Autodesk Inventor part; units mm, degrees
ref_plane "YZ Plane" through (0, 0, 0) normal (1, 0, 0) x (0, 1, 0)
ref_plane "XZ Plane" through (0, 0, 0) normal (0, 1, 0) x (-1, 0, 0)
ref_plane "XY Plane" through (0, 0, 0) normal (0, 0, 1) x (1, 0, 0)
sketch "Skizze1" plane through (0, 0, 0) normal (0, 0, 1) x (1, 0, 0)
  arc A0 (-10.0563, 3.3011) -> (-12.2178, -3.2473) centre (-1.2178, -3.2473) ccw
  line L0 (-12.2178, -3.2473) -> (9.7822, -3.2473)
  arc A1 (9.7822, -3.2473) -> (7.6207, 3.3011) centre (-1.2178, -3.2473) ccw
  arc A2 (-3.7041, 1.8719) -> (7.6207, 3.3011) centre (-1.2178, 27.7527) ccw
  line L1 (-3.7041, 1.8719) -> (-4.2446, 1.7527)
  line L2 (-4.2446, 1.7527) -> (-4.7816, 1.7527)
  line L3 (-4.7816, 1.7527) -> (-6.4898, 2.2928)
  arc A3 (-10.0563, 3.3011) -> (-6.4898, 2.2928) centre (-1.2178, 27.7527) ccw
  arc A4 (-12.2178, 58.7527) -> (-10.0563, 52.2043) centre (-1.2178, 58.7527) ccw
  arc A5 (7.6207, 52.2043) -> (-10.0563, 52.2043) centre (-1.2178, 27.7527) ccw
  arc A6 (7.6207, 52.2043) -> (9.7822, 58.7527) centre (-1.2178, 58.7527) ccw
  line L4 (9.7822, 58.7527) -> (-12.2178, 58.7527)
  line L5 (85.2075, 58.7527) -> (80.2075, 58.7527)
  line L6 (80.2075, 58.7527) -> (80.2075, 53.7527)
  line L7 (80.2075, 53.7527) -> (85.2075, 53.7527)
  line L8 (85.2075, 53.7527) -> (85.2075, 58.7527)
  line L9 (85.2075, -3.2473) -> (85.2075, 1.7527)
  line L10 (85.2075, 1.7527) -> (80.2075, 1.7527)
  line L11 (80.2075, 1.7527) -> (80.2075, -3.2473)
  line L12 (80.2075, -3.2473) -> (85.2075, -3.2473)
  circle A7 centre (19.8794, 52.7527) radius 3
  circle A8 centre (19.8794, 2.7527) radius 3
  circle A9 centre (-22.1206, 2.7527) radius 3
  circle A10 centre (-22.1206, 52.7527) radius 3
  line L13 (85.2075, 58.7527) -> (-62.1847, 58.7527)
  line L14 (-62.1847, 58.7527) -> (-62.1847, -3.2473)
  line L15 (-62.1847, -3.2473) -> (85.2075, -3.2473)
  line L16 (85.2075, -3.2473) -> (85.2075, 58.7527)
  point P0 (0, 0)
extrude "Extrusion1" add sketch "Skizze1" along normal blind 3
sketch "Skizze2" plane through (0, 0, 3) normal (0, 0, 1) x (1, 0, 0)
  circle A0 centre (-3.1206, 27.7527) radius 15
  line L0 (85.2075, 58.7527) -> (-62.1847, 58.7527)
  line L1 (-62.1847, -3.2473) -> (85.2075, -3.2473)
  line L2 (27.3951, 58.7527) -> (31.3951, 58.7527)
  line L3 (31.3951, 58.7527) -> (31.3951, -3.2473)
  line L4 (31.3951, -3.2473) -> (27.3951, -3.2473)
  line L5 (27.3951, -3.2473) -> (27.3951, 58.7527)
  line L6 (35.5129, 58.7527) -> (39.5129, 58.7527)
  line L7 (39.5129, 58.7527) -> (39.5129, 3.8427)
  line L8 (39.5129, 3.8427) -> (35.5129, 3.8427)
  line L9 (35.5129, 3.8427) -> (35.5129, 58.7527)
  line L10 (85.2075, -3.2473) -> (85.2075, 58.7527)
  line L11 (39.5129, 3.8427) -> (85.2075, 3.8427)
  line L12 (85.2075, 3.8427) -> (85.2075, 7.8427)
  line L13 (85.2075, 7.8427) -> (39.5129, 7.8427)
  line L14 (39.5129, 7.8427) -> (39.5129, 3.8427)
  line L15 (39.5129, 58.7527) -> (85.2075, 58.7527)
  line L16 (85.2075, 58.7527) -> (85.2075, 54.7527)
  line L17 (85.2075, 54.7527) -> (39.5129, 54.7527)
  line L18 (39.5129, 54.7527) -> (39.5129, 58.7527)
  point P0 (0, 0)
  dimension "d2" = 4
  dimension "d3" = 4
  dimension "d4" = 45.6946
  dimension "d5" = 4
  dimension "d12" = 45.6946
  dimension "d13" = 4
extrude "Extrusion2" add sketch "Skizze2" along normal blind 35 contours L10 L17 L7 L0 | L7 L8 L9 L0 | L10 L11 L7 L13 | L3 L1 L5 L0
sketch "Skizze3" plane through (0, 0, 3) normal (0, 0, 1) x (1, 0, 0)
  line L0 (39.5129, 54.7527) -> (39.5129, 7.8427)
  line L1 (39.5129, 7.8427) -> (85.2075, 7.8427)
  line L2 (85.2075, 7.8427) -> (85.2075, 54.7527)
  line L3 (35.5129, 58.7527) -> (31.3951, 58.7527)
  line L4 (27.7822, 53.7527) -> (85.2075, 53.7527)
  line L5 (39.5129, 7.8427) -> (85.2075, 7.8427)
  line L6 (85.2075, 7.8427) -> (85.2075, 53.7527)
  line L7 (85.2075, 53.7527) -> (39.5129, 53.7527)
  line L8 (39.5129, 53.7527) -> (39.5129, 7.8427)
  line L9 (35.5129, 3.8427) -> (35.5129, 58.7527)
  line L10 (31.3951, 58.7527) -> (31.3951, -3.2473)
  line L11 (31.3951, -3.2473) -> (85.2075, -3.2473)
  line L12 (85.2075, -3.2473) -> (85.2075, 3.8427)
  line L13 (85.2075, 3.8427) -> (35.5129, 3.8427)
  line L14 (85.2075, 54.7527) -> (39.5129, 54.7527)
  line L15 (27.3951, -3.2473) -> (27.3951, 58.7527)
  line L16 (27.3951, 58.7527) -> (-62.1847, 58.7527)
  line L17 (-62.1847, 58.7527) -> (-62.1847, -3.2473)
  line L18 (-62.1847, -3.2473) -> (27.3951, -3.2473)
  point P0 (0, 0)
extrude "Extrusion3" cut sketch "Skizze3" against normal blind 35 contours L4 L2 L1 L0
sketch "Skizze4" plane through (39.5129, 7.8427, 38) normal (1, 0, 0) x (0, 0, -1)
  line L0 (0, 0) -> (38, 0)
  line L1 (38, 45.91) -> (38, 0)
  line L2 (35, 45.91) -> (38, 45.91)
  line L3 (35, 46.91) -> (35, 45.91)
  line L4 (0, 0) -> (0, 46.91)
  line L5 (0, 0) -> (38, 0)
  line L6 (33.1404, 0) -> (3.7306, 0)
  line L7 (3.7306, 0) -> (3.7306, 42.1415)
  line L8 (3.7306, 42.1415) -> (33.1404, 42.1415)
  line L9 (33.1404, 42.1415) -> (33.1404, 0)
  line L10 (35, 46.91) -> (0, 46.91)
  point P0 (38, -7.8427)
extrude "Extrusion4" cut sketch "Skizze4" against normal blind 35 contours L7 L8 L9 L0
fillet "Rundung1" radius 35 2 edges at (85.2075, 5.8427, 38) (85.2075, 56.7527, 38)
sketch "Skizze5" plane through (-62.1847, 58.7527, 0) normal (0, 1, 0) x (1, 0, 0)
  arc A0 (112.3922, -38) -> (147.3922, -3) centre (112.3922, -3) ccw
  line L0 (147.3922, 0) -> (147.3922, -3)
  line L1 (147.3922, 0) -> (0, 0)
  line L2 (0, 0) -> (0, -3)
  line L3 (89.5798, -3) -> (0, -3)
  line L4 (89.5798, -3) -> (89.5798, -38)
  line L5 (93.5798, -38) -> (89.5798, -38)
  line L6 (93.5798, -3) -> (93.5798, -38)
  line L7 (97.6976, -3) -> (93.5798, -3)
  line L8 (97.6976, -3) -> (97.6976, -38)
  line L9 (112.3922, -38) -> (97.6976, -38)
  circle A1 centre (114.698, -22) radius 2.5
  point P0 (62.1847, 0)
  dimension "d15" = 5
extrude "Extrusion5" cut sketch "Skizze5" against normal through all contours A1
properties part number "13_Zwischenebene_LCD"
CAD build for the part. Positions are in the model's coordinates, mm. A direction names the side the tool comes from. Coordinates: 2 decimals unless noted, no trailing zeros. Write each loop counter-clockwise with the first axis right and the second up, starting at its lowest first coordinate (ties: lowest second). Pieces come first, ordered by that corner, then holes.
(1) 3-axis set-ups, long thin cutter, end or side, ignore diameter. For faces 1 (the face through (48, 3, 3)), 2 (the face through (55, 3.843, 20)), 3 (the face through (58, 54.753, 16)), 4 (the face through (29, 7.843, 20)), 5 (the face through (27.395, 20, 36)): which of +Z, -Z, +X, -X, +Y, -Y reach the whole face in a straight line?
(2) Two-plate mould, pull along Z, no slides. Class faces 6 (the face through (-22.51, 49.78, 1.48)), 7 (the face through (54.9, 5.87, 21.25)), 8 (the face through (29, 29, 34.269)), 9 (the face through (74.7, 56.8, 28)): +Z half, -Z half, draft (parallel to the pull), parting line (faces both ways), or undercut.
(3) Cut at B-B, the plane x = 48.5. List the corners of the cut face in (y, z).
(4) Cut at C-C, the plane z = 13. List the corners of the cut face in (x, y).
(5) Flat gauge pins, fed straight in: pin 1 (6 mm diameter, centred on y = 35.5, z = 4, fed in from +X); pin 2 (4 mm diameter, centred on x = 35, z = 11, fed in from -Y); pin 3 (12 mm diameter, centred on y = 26.5, z = 13, fed in from +X); pin 4 (7 mm diameter, centred on x = 19.88, y = 52.75, fed in from +Z). Where does each tip first touch, or does it go through?
(6) Cut at A-A, the plane y = 46.5. List the corners of the cut face in (x, z).
(7) Cut at D-D, the plane z = 22. List the corners of the cut face in (x, y).
(8) Drill centre lines: probe 1 along X at (y, z) = (15, 3.5); probe 2 along X at (y, z) = (56, 22); probe 3 along Y at (x, z) = (52, 28). Where is each one in solid material? Low to high.
Geometry says:
1. face 1: +Z, -Y
1. face 2: +Z, +X, -Y
1. face 3: +Z, +X
1. face 4: +X, -X
1. face 5: +Z, -X, +Y, -Y
2. face 6: draft
2. face 7: undercut
2. face 8: undercut
2. face 9: +Z half
3. outline: (-3.25, 0) - (7.84, 0) - (7.84, 38) - (3.84, 38) - (3.84, 3) - (-3.25, 3) - close; (53.75, 0) - (58.75, 0) - (58.75, 38) - (54.75, 38) - (54.75, 3) - (53.75, 3) - close
4. outline: (27.4, -3.25) - (31.4, -3.25) - (31.4, 7.84) - (27.4, 7.84) - close; (27.4, 49.98) - (31.4, 49.98) - (31.4, 58.75) - (27.4, 58.75) - close; (35.51, 3.84) - (83.75, 3.84) - (83.75, 7.84) - (35.51, 7.84) - close; (35.51, 49.98) - (39.51, 49.98) - (39.51, 54.75) - (83.75, 54.75) - (83.75, 58.75) - (35.51, 58.75) - close
5. pin 1: stops at x = 39.51
5. pin 2: stops at y = 3.84
5. pin 3: passes through
5. pin 4: stops at z = 3
6. outline: (-62.18, 0) - (39.51, 0) - (39.51, 4.86) - (35.51, 4.86) - (35.51, 3) - (31.4, 3) - (31.4, 4.86) - (27.4, 4.86) - (27.4, 3) - (-62.18, 3) - close; (27.4, 34.27) - (31.4, 34.27) - (31.4, 38) - (27.4, 38) - close; (35.51, 34.27) - (39.51, 34.27) - (39.51, 38) - (35.51, 38) - close
7. outline: (27.4, -3.25) - (31.4, -3.25) - (31.4, 7.84) - (27.4, 7.84) - close; (27.4, 49.98) - (31.4, 49.98) - (31.4, 58.75) - (27.4, 58.75) - close; (35.51, 3.84) - (50.01, 3.84) - (50.01, 7.84) - (35.51, 7.84) - close; (35.51, 49.98) - (39.51, 49.98) - (39.51, 54.75) - (50.01, 54.75) - (50.01, 58.75) - (35.51, 58.75) - close; (55.01, 3.84) - (79.6, 3.84) - (79.6, 7.84) - (55.01, 7.84) - close; (55.01, 54.75) - (79.6, 54.75) - (79.6, 58.75) - (55.01, 58.75) - close
8. probe 1: x = 27.4 to 31.4, 35.51 to 39.51
8. probe 2: x = 27.4 to 31.4, 35.51 to 50.01, 55.01 to 79.6
8. probe 3: y = 3.84 to 7.84, 54.75 to 58.75
